from build123d import *

# Parameters (mm, degrees)
SKETCH_1_W          = 50
SKETCH_1_H          = 26
EXTRUDE_1_DEPTH     = 3
EXTRUDE_2_DEPTH     = 6
SKETCH_5_W          = 0.1
SKETCH_5_H          = 0.1
CUT_EXTRUDE_1_DEPTH = 3
SKETCH_4_W          = 3
SKETCH_4_H          = 26
EXTRUDE_7_DEPTH     = 103
SKETCH_6_W          = 3
SKETCH_6_H          = 26
EXTRUDE_8_DEPTH     = 50
EXTRUDE_9_DEPTH     = 3
SKETCH_9_W          = 6
SKETCH_9_H          = 53
EXTRUDE_12_DEPTH    = 3
SKETCH_10_R         = 1.7
CUT_EXTRUDE_2_DEPTH = 108.930533215


with BuildPart() as part:
    # 草图1 → 凸台-拉伸1 (new body)
    with BuildSketch(Plane(origin=(0, 0, 0), x_dir=(0, 0, -1), z_dir=(1, 0, 0))):
        Rectangle(SKETCH_1_W, SKETCH_1_H)
    extrude(amount=EXTRUDE_1_DEPTH)

    # 草图2 → 凸台-拉伸2 (add)
    with BuildSketch(Plane(origin=(3, 0, 0), x_dir=(0, 0, -1), z_dir=(1, 0, 0))):
        Polygon((-25, -13), (-17, -13), (-17, -7), align=None)
        Polygon((-8, -7), (-16, -13), (-8, -13), align=None)
        Polygon((1, -7), (-7, -13), (1, -13), align=None)
        Polygon((10, -7), (2, -13), (10, -13), align=None)
        Polygon((19, -7), (11, -13), (19, -13), align=None)
    extrude(amount=-EXTRUDE_2_DEPTH)

    # 草图5 → 切除-拉伸1 (cut)
    with BuildSketch(Plane.ZY):
        with Locations((25, -13)):
            Rectangle(SKETCH_5_W, SKETCH_5_H)
    extrude(amount=CUT_EXTRUDE_1_DEPTH, mode=Mode.SUBTRACT)

    # 草图4 → 凸台-拉伸7 (add)
    with BuildSketch(Plane(origin=(3, 0, 0), x_dir=(0, 0, -1), z_dir=(1, 0, 0))):
        with Locations((-26.5, 0)):
            Rectangle(SKETCH_4_W, SKETCH_4_H)
    extrude(amount=-EXTRUDE_7_DEPTH)

    # 草图6 → 凸台-拉伸8 (add, through all)
    with BuildSketch(Plane(origin=(0, 0, 25), x_dir=(-1, 0, 0), z_dir=(0, 0, -1))):
        with Locations((98.5, 0)):
            Rectangle(SKETCH_6_W, SKETCH_6_H)
    extrude(amount=EXTRUDE_8_DEPTH)

    # 草图7 → 凸台-拉伸9 (add)
    with BuildSketch(Plane(origin=(-97, 0, 0), x_dir=(0, 0, -1), z_dir=(1, 0, 0))):
        Polygon((-25, -7), (-25, -13), (-17, -13), align=None)
        Polygon((-8, -13), (-16, -7), (-16, -13), align=None)
        Polygon((1, -13), (-7, -7), (-7, -13), align=None)
        Polygon((10, -13), (2, -7), (2, -13), align=None)
        Polygon((19, -13), (11, -7), (11, -13), align=None)
    extrude(amount=EXTRUDE_9_DEPTH)

    # 草图9 → 凸台-拉伸12 (add)
    with BuildSketch(Plane(origin=(0, -13, 0), x_dir=(-1, 0, 0), z_dir=(0, -1, 0))):
        with Locations((0, -1.5)):
            Rectangle(SKETCH_9_W, SKETCH_9_H)
        with Locations((97, -1.5)):
            Rectangle(SKETCH_9_W, SKETCH_9_H)
    extrude(amount=EXTRUDE_12_DEPTH)

    # 草图10 → 切除-拉伸2 (cut, through all)
    with BuildSketch(Plane(origin=(3, 0, 0), x_dir=(0, 0, -1), z_dir=(1, 0, 0))):
        with Locations((20, 10)):
            Circle(SKETCH_10_R)
        with Locations((0, 10)):
            Circle(SKETCH_10_R)
    extrude(amount=-CUT_EXTRUDE_2_DEPTH, mode=Mode.SUBTRACT)


solid = part.part
Geometry: final body of the model. Coordinates: model frame, mm. A direction names the side the tool comes from. Round coordinates to 2 decimals unless told otherwise and drop trailing zeros. Loops run counter-clockwise (first coordinate to the right, second up) from the corner with the lowest first, then second, coordinate; pieces in that order, holes last. Notation, with made-up numbers: (6.5, 32.25) -> (57.5, 32.25) arc R16 cw to (57.5, 57.25) -> close; hole circle Ø6 at (22.25, 72.5). An arc over 180 degrees is marked (long way). One line per question, with ' | ' between items. Start each with the question number.
1. Section C-C on y = -3.75. Output: boundary loops of the cut face in (x, z).
2. Section B-B on z = -17. Output: boundary loops of the cut face in (x, y), and give its area (3 significant figures).
3. Section A-A on y = 10. Output: boundary loops of the cut face in (x, z).
4. Section D-D on z = 0. Output: boundary loops of the cut face in (x, y).
5. Contact query for flat-ended pins moving along their axis: pin 1 (3.5 mm diameter, centred on x = -1, y = -11, fed in from -Z); pin 2 (1 mm diameter, centred on x = -29, y = -6, fed in from -Z); pin 3 (0.9 mm diameter, centred on x = -1, y = -11.5, fed in from -Z); pin 4 (0.9 mm diameter, centred on x = -2, z = -22.5, fed in from +Y). Output: stop coordinate, or through.
6. Set-up query: faces 5 (the face through (1.52, 8.34, 0.37)), 6 (the face through (-1, -13, -22)), 7 (the face through (-49, -13, 27)), 8 (the face through (-96, -10, 7)), 9 (the face through (1, -1, -25)). Return all of +Z, -Z, +X, -X, +Y, -Y with unobstructed straight access to the full face (end or side cutting, diameter ignored); none if empty.
7. Line query: line 1 along X through (y, z) = (-2.25, -12); line 2 along Y through (x, z) = (1.85, 0); line 3 along X through (y, z) = (-12.5, -3.5). Output: solid intervals per line, ascending. Write a range as [from, to].
8. Mould query, pull axis Z, two halves, no side actions, for faces 1 (the face through (-98, -1, -25)), 2 (the face through (-1, -10, -15)), 3 (the face through (0, -16, 1)), 4 (the face through (-1, -10, 21)). Classes: pulls with the +Z half, pulls with the -Z half, needs draft (parallel to the pull), parting line crosses it, or undercut.
Returned:
1) outline: (-100, -25) -> (-97, -25) -> (-97, 25) -> (0, 25) -> (0, -25) -> (3, -25) -> (3, 28) -> (-100, 28) -> close
2) outline: (-100, -16) -> (-94, -16) -> (-94, -11.5) -> (-97, -11.5) -> (-97, 13) -> (-100, 13) -> close; (-3, -16) -> (3, -16) -> (3, 13) -> (0, 13) -> (0, -8.5) -> (-3, -8.5) -> close | area: 210 mm2
3) outline: (-100, -25) -> (-97, -25) -> (-97, -21.7) -> (-100, -21.7) -> close; (-100, -18.3) -> (-97, -18.3) -> (-97, -1.7) -> (-100, -1.7) -> close; (-100, 1.7) -> (-97, 1.7) -> (-97, 25) -> (0, 25) -> (0, 1.7) -> (3, 1.7) -> (3, 28) -> (-100, 28) -> close; (0, -25) -> (3, -25) -> (3, -21.7) -> (0, -21.7) -> close; (0, -18.3) -> (3, -18.3) -> (3, -1.7) -> (0, -1.7) -> close
4) outline: (-100, -16) -> (-94, -16) -> (-94, -12.25) -> (-97, -12.25) -> (-97, 8.3) -> (-100, 8.3) -> close; (-100, 11.7) -> (-97, 11.7) -> (-97, 13) -> (-100, 13) -> close; (-3, -16) -> (3, -16) -> (3, 8.3) -> (0, 8.3) -> (0, -7.75) -> (-3, -7.75) -> close; (0, 11.7) -> (3, 11.7) -> (3, 13) -> (0, 13) -> close
5) pin 1: stops at z = -25 | pin 2: stops at z = 25 | pin 3: stops at z = -19 | pin 4: stops at y = -13
6) face 5: +X, -X | face 6: -Z, +Y | face 7: +Z, -Z, -Y | face 8: +Y | face 9: -Z, +X, -X, +Y, -Y
7) line 1: x = [-100, -97], [0, 3] | line 2: y = [-16, 8.3], [11.7, 13] | line 3: x = [-100, -94], [-3, 3]
8) face 1: pulls with the -Z half | face 2: undercut | face 3: needs draft | face 4: undercut
